```python
from build123d import *

# Parameters (mm, degrees)
F0_W     = 2
F0_H     = 19
F0_H_2   = 16
F0_W_2   = 18.0994240791
F0_H_3   = 2
F0_H_4   = 1
F0_H_5   = 23.25
F0_H_6   = 13
F0_H_7   = 6
F0_W_3   = 10
F0_H_8   = 5.75
F1_DEPTH = 3
F2_DEPTH = 4.5
F3_DEPTH = 11
F5_DEPTH = 4.5
F6_DEPTH = 4.5
F7_DEPTH = 4.5


# Not quite as in the source:
# - a feature names something its author has since deleted; it is built from what else it names


with BuildPart() as f1:
    # F0 (on Top) → F1 (new body)
    with BuildSketch(Plane.XY):
        Polygon((-48.8793104887, -18.5732776225), (-48.8793104887, 0.4267223775), (-46.8793104887, 0.4267223775), (9.0212654322, 0.4267223775), (27.1206895113, 0.4267223775), (29.1206895113, 0.4267223775), (29.1206895113, 6.4267223775), (-50.8793104887, 6.4267223775), (-50.8793104887, -1.5732776225), (-50.8793104887, -18.5732776225), align=None)
        with Locations((-47.8793104887, -9.0732776225)):
            Rectangle(F0_W, F0_H)
        Polygon((9.0212654322, 0.4267223775), (-46.8793104887, 0.4267223775), (-46.8793104887, -18.5732776225), (-46.8793104887, -34.5732776225), (-46.8793104887, -35.5732776225), (9.6206895113, -35.5732776225), (19.6206895113, -35.5732776225), (27.1206895113, -35.5732776225), (27.1206895113, -1.5732776225), (9.0212654322, -1.5732776225), align=None)
        with Locations((-47.8793104887, -26.5732776225)):
            Rectangle(F0_W, F0_H_2)
        with Locations((18.0709774718, -0.5732776225)):
            Rectangle(F0_W_2, F0_H_3)
        with Locations((-47.8793104887, -35.0732776225)):
            Rectangle(F0_W, F0_H_4)
        Polygon((-48.8793104887, -35.5732776225), (-48.8793104887, -34.5732776225), (-50.8793104887, -34.5732776225), (-50.8793104887, -35.5732776225), (-50.8793104887, -41.5732776225), (27.1206895113, -41.5732776225), (27.1206895113, -35.5732776225), (19.6206895113, -35.5732776225), (19.6206895113, -37.5732776225), (9.6206895113, -37.5732776225), (9.6206895113, -35.5732776225), (-46.8793104887, -35.5732776225), align=None)
        Polygon((29.1206895113, 0.4267223775), (27.1206895113, 0.4267223775), (27.1206895113, -1.5732776225), (27.1206895113, -35.5732776225), (29.1206895113, -35.8232776225), (29.1206895113, -22.8232776225), align=None)
        with Locations((30.1206895113, -11.1982776225)):
            Rectangle(F0_W, F0_H_5)
        Polygon((29.1206895113, 6.4267223775), (29.1206895113, 0.4267223775), (31.1206895113, 0.4267223775), (31.1206895113, 6.4267223775), (30.1206895113, 6.4267223775), align=None)
        with Locations((30.1206895113, -29.3232776225)):
            Rectangle(F0_W, F0_H_6)
        with Locations((32.1206895113, -11.1982776225)):
            Rectangle(F0_W, F0_H_5)
        with Locations((32.1206895113, 3.4267223775)):
            Rectangle(F0_W, F0_H_7)
        Polygon((29.1206895113, -35.8232776225), (27.1206895113, -35.5732776225), (27.1206895113, -41.5732776225), (29.1206895113, -41.5732776225), align=None)
        with Locations((14.6206895113, -36.5732776225)):
            Rectangle(F0_W_3, F0_H_3)
        Polygon((31.1206895113, -35.8232776225), (29.1206895113, -35.8232776225), (29.1206895113, -41.5732776225), (30.1206895113, -41.5732776225), (31.1206895113, -41.5732776225), align=None)
        with Locations((32.1206895113, -29.3232776225)):
            Rectangle(F0_W, F0_H_6)
        with Locations((32.1206895113, -38.6982776225)):
            Rectangle(F0_W, F0_H_8)
    extrude(amount=-F1_DEPTH)

    # F0 (on Top) → F2 (join)
    with BuildSketch(Plane.XY):
        with Locations((-47.8793104887, -9.0732776225)):
            Rectangle(F0_W, F0_H)
        with Locations((-47.8793104887, -26.5732776225)):
            Rectangle(F0_W, F0_H_2)
        with Locations((18.0709774718, -0.5732776225)):
            Rectangle(F0_W_2, F0_H_3)
        with Locations((-47.8793104887, -35.0732776225)):
            Rectangle(F0_W, F0_H_4)
    extrude(amount=F2_DEPTH)

    # F0 (on Top) → F3 (join)
    with BuildSketch(Plane.XY):
        Polygon((-48.8793104887, -18.5732776225), (-48.8793104887, 0.4267223775), (-46.8793104887, 0.4267223775), (9.0212654322, 0.4267223775), (27.1206895113, 0.4267223775), (29.1206895113, 0.4267223775), (29.1206895113, 6.4267223775), (-50.8793104887, 6.4267223775), (-50.8793104887, -1.5732776225), (-50.8793104887, -18.5732776225), align=None)
        with Locations((-47.8793104887, -9.0732776225)):
            Rectangle(F0_W, F0_H)
        with Locations((18.0709774718, -0.5732776225)):
            Rectangle(F0_W_2, F0_H_3)
        Polygon((-48.8793104887, -35.5732776225), (-48.8793104887, -34.5732776225), (-50.8793104887, -34.5732776225), (-50.8793104887, -35.5732776225), (-50.8793104887, -41.5732776225), (27.1206895113, -41.5732776225), (27.1206895113, -35.5732776225), (19.6206895113, -35.5732776225), (19.6206895113, -37.5732776225), (9.6206895113, -37.5732776225), (9.6206895113, -35.5732776225), (-46.8793104887, -35.5732776225), align=None)
        with Locations((30.1206895113, -11.1982776225)):
            Rectangle(F0_W, F0_H_5)
        Polygon((29.1206895113, 6.4267223775), (29.1206895113, 0.4267223775), (31.1206895113, 0.4267223775), (31.1206895113, 6.4267223775), (30.1206895113, 6.4267223775), align=None)
        with Locations((32.1206895113, -11.1982776225)):
            Rectangle(F0_W, F0_H_5)
        with Locations((32.1206895113, 3.4267223775)):
            Rectangle(F0_W, F0_H_7)
        Polygon((29.1206895113, -35.8232776225), (27.1206895113, -35.5732776225), (27.1206895113, -41.5732776225), (29.1206895113, -41.5732776225), align=None)
        Polygon((31.1206895113, -35.8232776225), (29.1206895113, -35.8232776225), (29.1206895113, -41.5732776225), (30.1206895113, -41.5732776225), (31.1206895113, -41.5732776225), align=None)
        with Locations((32.1206895113, -38.6982776225)):
            Rectangle(F0_W, F0_H_8)
    extrude(amount=F3_DEPTH)

    # F4 (on face) → F5 (join)
    with BuildSketch(Plane.XY.offset(11)):
        Polygon((22.1148194903, -35.5732776225), (19.6206895113, -35.5732776225), (19.6206895113, -37.5732776225), (9.6206895113, -37.5732776225), (9.6206895113, -35.5732776225), (-48.8793104887, -35.5732776225), (-48.8793104887, -37.5732776225), (7.6206895113, -37.5732776225), (7.6206895113, -39.5732776225), (21.6206895113, -39.5732776225), (21.6206895113, -36.236452068), align=None)
    extrude(amount=F5_DEPTH)

    # F0 (on Top) → F6 (join)
    with BuildSketch(Plane.XY):
        Polygon((29.1206895113, 0.4267223775), (27.1206895113, 0.4267223775), (27.1206895113, -1.5732776225), (27.1206895113, -35.5732776225), (29.1206895113, -35.8232776225), (29.1206895113, -22.8232776225), align=None)
    extrude(amount=F6_DEPTH)

    # F4 (on face) → F7 (join)
    with BuildSketch(Plane.XY.offset(11)):
        Polygon((31.1206895113, -22.8232776225), (31.1206895113, 2.4267223775), (29.1206895113, 2.4267223775), (-48.8793104887, 2.4267223775), (-48.8793104887, -18.5732776225), (-46.8793104887, -18.5732776225), (-46.8793104887, 0.4267223775), (29.1206895113, 0.4267223775), (29.1206895113, -22.8232776225), align=None)
    extrude(amount=F7_DEPTH)


solid = f1.part
```
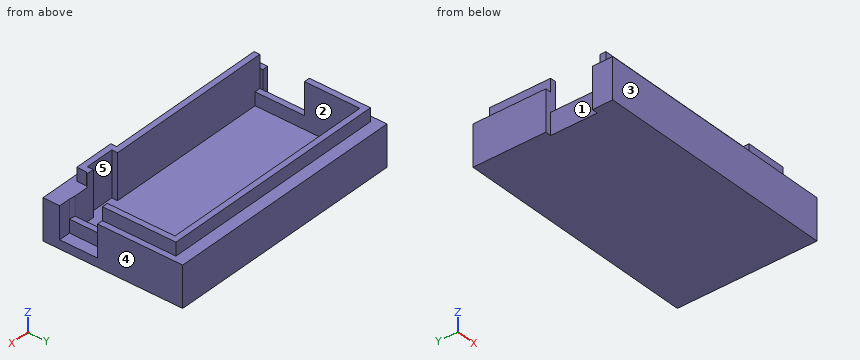
The listing builds one solid part. Answer for the finished solid, in the listing's coordinates (mm). Face numbers are marked on the shaded views. A direction names the side the tool comes from. Give positions to 0.01 mm unless a question says otherwise; leave off trailing zeros. Write each loop counter-clockwise with the first axis right and the second up, starting at its lowest first coordinate (ties: lowest second). Pieces come first, ordered by that corner, then holes. Notation, with made-up numbers: (80, 46.5) -> (120, 46.5) arc R31 ccw to (120, 82.5) -> close; hole circle Ø10 at (44, 36.5). An arc over 180 degrees is marked (long way). Use one line per item in the form item = value.
1) Each of these flat-tipped pins is pushed along its axis until it touches: P1, Ø0.6, axis at x = 22, y = -0.5, coming from the +Z side; P2, Ø2, axis at y = -25, z = 0, coming from the -X side; P3, Ø12, axis at x = 17, y = -16, coming from the +Z side. Where does it stop, or does it pass through?
Result:
P1 = 11
P2 = -48.88
P3 = 0
2) Section B-B on y = -24 is taken. Write down the section's boundary in (x, z), plus the area to 3 significant figures.
Result:
outline = (-48.88, -3) -> (33.12, -3) -> (33.12, 0) -> (29.12, 0) -> (29.12, 4.5) -> (27.12, 4.5) -> (27.12, 0) -> (-46.88, 0) -> (-46.88, 4.5) -> (-48.88, 4.5) -> close
area = 264 mm²
3) Section C-C on z = 1.5 is taken. Write down the section's boundary in (x, y), plus the area to 3 significant figures.
Result:
outline = (-50.88, -41.57) -> (33.12, -41.57) -> (33.12, -35.82) -> (29.12, -35.82) -> (29.12, -22.82) -> (33.12, -22.82) -> (33.12, 6.43) -> (-50.88, 6.43) -> (-50.88, -18.57) -> (-48.88, -18.57) -> (-48.88, -34.57) -> (-50.88, -34.57) -> close; hole (-46.88, -35.57) -> (9.62, -35.57) -> (9.62, -37.57) -> (19.62, -37.57) -> (19.62, -35.57) -> (27.12, -35.57) -> (27.12, -1.57) -> (9.02, -1.57) -> (9.02, 0.43) -> (-46.88, 0.43) -> close
area = 1,300 mm²
4) For a pull along X with two mould halves and no side action, classify the marked faces 1, 2 and 3 as +X half, -X half, draft (parallel to the pull), parting line (faces both ways), or undercut.
Result:
face_1 = -X half
face_2 = undercut
face_3 = draft
5) Section A-A on z = 13 is taken. Write down the section's boundary in (x, y).
Result:
outline = (-48.88, -37.57) -> (7.62, -37.57) -> (7.62, -39.57) -> (21.62, -39.57) -> (21.62, -36.24) -> (22.11, -35.57) -> (19.62, -35.57) -> (19.62, -37.57) -> (9.62, -37.57) -> (9.62, -35.57) -> (-48.88, -35.57) -> close; (-48.88, -18.57) -> (-46.88, -18.57) -> (-46.88, 0.43) -> (29.12, 0.43) -> (29.12, -22.82) -> (31.12, -22.82) -> (31.12, 2.43) -> (-48.88, 2.43) -> close
6) A tool of negligible diameter and unlimited length cuts with its end or side. For the marked faces 4 and 5, from which of +Z, -Z, +X, -X, +Y, -Y can it reach the whole face along a straight path? Write none if from no direction.
Result:
face_4 = +Z, -Z, +X, +Y, -Y
face_5 = +Z
7) Section D-D on x = -17.5 is taken. Write down the section's boundary in (y, z), plus the area to 3 significant figures.
Result:
outline = (-41.57, -3) -> (6.43, -3) -> (6.43, 11) -> (2.43, 11) -> (2.43, 15.5) -> (0.43, 15.5) -> (0.43, 0) -> (-35.57, 0) -> (-35.57, 15.5) -> (-37.57, 15.5) -> (-37.57, 11) -> (-41.57, 11) -> close
area = 294 mm²
8) Straight lines are drawn through the part: probe 1 along Y at (x, z) = (-45.5, 5); probe 2 along X at (y, z) = (-10, 1.5); probe 3 along Y at (x, z) = (13.5, 4). For each, find the intervals that lie inside material, in ascending order.
Result:
probe_1 = -41.57 to -35.57, 0.43 to 6.43
probe_2 = -50.88 to -46.88, 27.12 to 33.12
probe_3 = -41.57 to -37.57, -1.57 to 6.43
